Read the model definition and answer for the solid it produces. Units are mm, in the model's axes. Face numbers are marked on the shaded views. A direction names the side the tool comes from. Round coordinates to 2 decimals unless told otherwise and drop trailing zeros. Loops run counter-clockwise (first coordinate to the right, second up) from the corner with the lowest first, then second, coordinate; pieces in that order, holes last. Notation, with made-up numbers: (24, 64.5) - (43, 64.5) arc R32 ccw to (43, 99.5) - close; hole circle Ø8 at (24, -39.75). An arc over 180 degrees is marked (long way). Use CSV: the item, a comma, the result in double quotes. Start each with the question number.
1. Given pin 1 Ø10.5 at (x, y) = (-0.5, -9) entering from +Z; pin 2 Ø1 at (y, z) = (22, 13) entering from -X; pin 3 Ø2 at (y, z) = (-1, 26.5) entering from +X, each flat-ended and moving along its own axis, determine where each tip first touches the part or whether it passes through.
2. Find section C-C (z = 8.5). Give the vertices of the cut face in (x, y), and give its area (3 significant figures).
3. Consider line 1 along Y through (x, z) = (-2.5, 21); line 2 along Y through (x, z) = (-20.5, 39); line 3 along Y through (x, z) = (8, 30). Determine where each line is inside the solid, lowest interval first.
4. Find section A-A (z = 25.5). Give the vertices of the cut face in (x, y), and give its area (3 significant figures).
5. Determine the mould class of the marked faces 4, 5 and 6 for opening direction Y: +Y half, -Y half, draft (parallel to the pull), parting line (faces both ways), or undercut.
6. A tool of negligible diameter and unlimited length cuts with its end or side. For the marked faces 1, 2 and 3, from which of +Z, -Z, +X, -X, +Y, -Y can it reach the whole face along a straight path? Write none if from no direction.
7. Find section B-B (z = 3). Give the vertices of the cut face in (x, y).
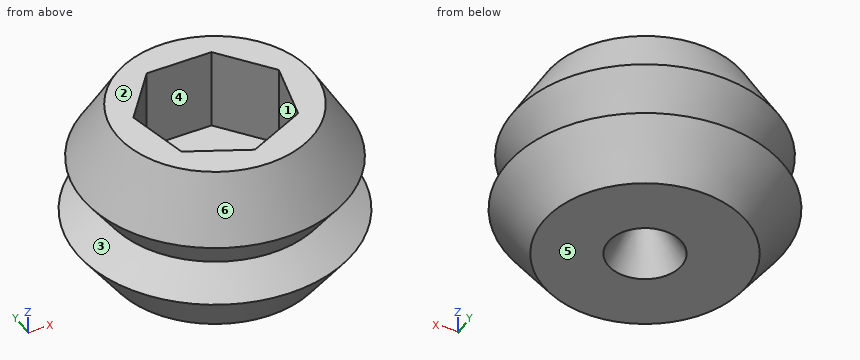
from build123d import *

# Parameters (mm, degrees)
F3_DEPTH = 20


with BuildPart() as f1:
    # F0 (on Front) → F1 (revolve)
    with BuildSketch(Plane.XZ):
        Polygon((-8.977577, 0), (0, 16.091861), (0, 40.822521), (-23.88373, 40.822521), (-32.302976, 26.567327), (-25.935675, 17.91742), (-33.708245, 12.195937), (-24.730667, 0), align=None)
    revolve(axis=Axis((0, 0, 28.457191), (0, 0, -1)))

    # F2 (on face) → F3 (cut)
    with BuildSketch(Plane.XY.offset(40.822521)):
        Polygon((7.907405, 16.419895), (-7.907405, 16.419895), (-17.767777, 4.055379), (-14.248651, -11.36292), (0, -18.224709), (14.248651, -11.36292), (17.767777, 4.055379), align=None)
    extrude(amount=-F3_DEPTH, mode=Mode.SUBTRACT)


solid = f1.part
Filled sheet:
1,pin 1,"stops at z = 20.82"
1,pin 2,"stops at x = -25.09"
1,pin 3,"stops at x = 32.3"
2,outline,"circle Ø61.98 at (0, 0); hole circle Ø8.47 at (0, 0)"
2,area,"2,960 mm²"
3,line 1,"y = -28.09 to -17.02, 16.42 to 28.09"
3,line 2,"y = -14.24 to 14.24"
3,line 3,"y = -29.2 to -14.37, 16.3 to 29.2"
4,outline,"circle Ø63.03 at (0, 0); hole (-17.77, 4.06) - (-14.25, -11.36) - (0, -18.22) - (14.25, -11.36) - (17.77, 4.06) - (7.91, 16.42) - (-7.91, 16.42) - close"
4,area,"2,210 mm²"
5,face 4,"undercut"
5,face 5,"draft"
5,face 6,"parting line"
6,face 1,"+Z"
6,face 2,"+Z, +X, -X, +Y, -Y"
6,face 3,"none"
7,outline,"circle Ø53.88 at (0, 0); hole circle Ø14.61 at (0, 0)"
